Part model, mm, in its own coordinate system. A direction names the side the tool comes from. Give positions to 0.01 mm unless a question says otherwise; leave off trailing zeros. Order: outer loops, then holes, each group sorted by start corner. A loop starts at its lowest first (then second) coordinate and runs counter-clockwise, first axis right, second up. Notation, with made-up numbers: M 87.25,1 L 132.25,1 A20 ccw 132.25,33 Z; hole C 45.5,73 d5. An arc over 180 degrees is marked long. Answer as a JSON object with one key per item and string values.
from build123d import *

# Parameters (mm, degrees)
F0_W     = 8.9916
F0_H     = 10.4902
F1_DEPTH = 9.398
F2_R     = 2.99
F3_DEPTH = 3.6068
F4_W     = 2.0066
F4_H     = 1.27
F5_DEPTH = 5.207
F6_W     = 2.0066
F6_H     = 1.27
F7_DEPTH = 5.9944


with BuildPart() as f1:
    # F0 (on Top) → F1 (new body)
    with BuildSketch(Plane.XY):
        Rectangle(F0_W, F0_H)
    extrude(amount=F1_DEPTH)

    # F2 (on face) → F3 (join)
    with BuildSketch(Plane.XY.offset(9.398)):
        Circle(F2_R)
    extrude(amount=F3_DEPTH)

    # F4 (on face) → F5 (join)
    with BuildSketch(Plane(origin=(0, 5.2451, 0), x_dir=(-1, 0, 0), z_dir=(0, 1, 0))):
        with Locations((0, 8.763)):
            Rectangle(F4_W, F4_H)
    extrude(amount=F5_DEPTH)

    # F6 (on face) → F7 (join)
    with BuildSketch(Plane(origin=(0, 0, 0), x_dir=(1, 0, 0), z_dir=(0, 0, -1))):
        with Locations((0, 4.6101)):
            Rectangle(F6_W, F6_H)
        with Locations((0, -4.6101)):
            Rectangle(F6_W, F6_H)
    extrude(amount=F7_DEPTH)


solid = f1.part
1. Cut at A-A on x = 0. Give the cut face in (y, z).
Worked answers:
{"outline": "M -5.25,-5.99 L -3.98,-5.99 L -3.98,0 L 3.98,0 L 3.98,-5.99 L 5.25,-5.99 L 5.25,8.13 L 10.45,8.13 L 10.45,9.4 L 2.99,9.4 L 2.99,13 L -2.99,13 L -2.99,9.4 L -5.25,9.4 Z"}
2. Probe line 1 along Y through (x, z) = (4, 1); line 2 along Z through (x, y) = (2, -0.5); line 3 along Z through (x, y) = (-0.5, 9.25). List the from-to ranges inside material, lowest first.
Worked answers:
{"line 1": "y = -5.25 to 5.25", "line 2": "z = 0 to 13", "line 3": "z = 8.13 to 9.4"}
3. Two-plate mould, pull along Y, no slides. Class faces 6 (the flat face through (-1.003, -5, -3)), 7 (the flat face through (0, 3.975, -3)), 8 (the flat face through (0, -3.975, -3)), 9 (the flat face through (0, -5.245, 3)): +Y half, -Y half, draft (parallel to the pull), parting line (faces both ways), or undercut.
Worked answers:
{"face 6": "draft", "face 7": "undercut", "face 8": "undercut", "face 9": "-Y half"}
4. Which spindle directions (+Z, -Z, +X, -X, +Y, -Y) get a long thin tool onto all of the face, cutting with end or side? Do faces 1 (the flat face through (0, 8, 8.128)), 2 (the flat face through (-1.003, 8, 9)), 3 (the flat face through (1.003, -5, -3)), 4 (the flat face through (-1.003, 5, -3)), 5 (the flat face through (2, 3, 9.398)). Say none if no direction does.
Worked answers:
{"face 1": "-Z, +X, -X, +Y", "face 2": "+Z, -Z, -X, +Y", "face 3": "-Z, +X, +Y, -Y", "face 4": "-Z, -X, +Y, -Y", "face 5": "+Z"}
5. Pin check, flat tips, straight feed: P1, Ø4.5, axis at x = 1, z = 5.5, coming from the +Y side; P2, Ø1.4, axis at y = 8, z = 9, coming from the -X side; P3, Ø8, axis at y = 7, z = 2, coming from the +X side; P4, Ø1, axis at y = 4.5, z = -4.5, coming from the +X side. Stop position of each tip, or through.
Worked answers:
{"P1": "stops at y = 5.25", "P2": "stops at x = -1", "P3": "stops at x = 4.5", "P4": "stops at x = 1"}
6. Cut at B-B on y = 4.5. Give the cut face in (x, z).
Worked answers:
{"outline": "M -4.5,0 L -1,0 L -1,-5.99 L 1,-5.99 L 1,0 L 4.5,0 L 4.5,9.4 L -4.5,9.4 Z"}
7. Cut at C-C on z = 3. Give the cut face in (x, y).
Worked answers:
{"outline": "M -4.5,-5.25 L 4.5,-5.25 L 4.5,5.25 L -4.5,5.25 Z"}
8. Cut at D-D on y = 0. Give the cut face in (x, z).
Worked answers:
{"outline": "M -4.5,0 L 4.5,0 L 4.5,9.4 L 2.99,9.4 L 2.99,13 L -2.99,13 L -2.99,9.4 L -4.5,9.4 Z"}
